Source: CAD feature listing. Evaluate the final solid. Frame: model axes, mm. A direction names the side the tool comes from. Coordinates: 2 decimals unless noted, no trailing zeros. Order: outer loops, then holes, each group sorted by start corner. A loop starts at its lowest first (then second) coordinate and runs counter-clockwise, first axis right, second up.
```python
from build123d import *

# Parameters (mm, degrees)
SKETCH1_W           = 340
SKETCH1_H           = 198
BOSS_EXTRUDE1_DEPTH = 22


with BuildPart() as part:
    # Sketch1 → Boss-Extrude1 (new body)
    with BuildSketch(Plane.XY):
        Polygon((-217.5, 109), (217.5, 109), (217.5, 99), (180, 99), (180, -109), (-180, -109), (-180, 99), (-217.5, 99), align=None)
        Rectangle(SKETCH1_W, SKETCH1_H, mode=Mode.SUBTRACT)
    extrude(amount=BOSS_EXTRUDE1_DEPTH)


solid = part.part
```
1. Section query C-C on y = -17. Return loops of the section in (x, z), plus the area to 3 significant figures.
Findings:
outline: (-180, 0) - (-170, 0) - (-170, 22) - (-180, 22) - close; (170, 0) - (180, 0) - (180, 22) - (170, 22) - close
area: 440 mm2
2. Access query for faces 1 (the face through (-198, 99, 11)), 2 (the face through (180, -4, 11)), 3 (the face through (170, -1, 11)), 4 (the face through (217.5, 104, 11)). Directions: +Z, -Z, +X, -X, +Y, -Y. A direction counts if a zero-diameter tool reaches every point of the face in a straight line with its end or side. Return the directions, or none.
Findings:
face 1: +Z, -Z, -X, -Y
face 2: +Z, -Z, +X, -Y
face 3: +Z, -Z
face 4: +Z, -Z, +X, +Y, -Y
3. Pin query (flat end, axial travel): P1, Ø11, axis at x = 192.5, z = 9.5, coming from the -Y side; P2, Ø4, axis at y = 73, z = 13.5, coming from the +X side; P3, Ø4, axis at y = 11.5, z = 14, coming from the -X side. Return the tip coordinate at first contact, or that it passes through.
Findings:
P1: stops at y = 99
P2: stops at x = 180
P3: stops at x = -180
4. Draft query along Y for faces 5 (the face through (-2, 99, 11)), 6 (the face through (3, -109, 11)), 7 (the face through (-217.5, 104, 11)). Return one class per face: released by +Y, released by -Y, zero draft, split by the parting line, or undercut.
Findings:
face 5: undercut
face 6: released by -Y
face 7: zero draft
5. Section query B-B on z = 6. Return loops of the section in (x, y), plus the area to 3 significant figures.
Findings:
outline: (-217.5, 99) - (-180, 99) - (-180, -109) - (180, -109) - (180, 99) - (217.5, 99) - (217.5, 109) - (-217.5, 109) - close; hole (-170, -99) - (170, -99) - (170, 99) - (-170, 99) - close
area: 11,900 mm2
6. Section query D-D on x = -187. Return loops of the section in (y, z).
Findings:
outline: (99, 0) - (109, 0) - (109, 22) - (99, 22) - close
7. Section query A-A on x = 51.5. Return loops of the section in (y, z), plus the area to 3 significant figures.
Findings:
outline: (-109, 0) - (-99, 0) - (-99, 22) - (-109, 22) - close; (99, 0) - (109, 0) - (109, 22) - (99, 22) - close
area: 440 mm2
8. Ray query, line 1 (X direction, y = 20.5, z = 18); line 2 (Y direction, x = -123.5, z = 6.5); line 3 (Y direction, x = -187, z = 15.5). Return the intervals inside material, ascending.
Findings:
line 1: x = -180 to -170, 170 to 180
line 2: y = -109 to -99, 99 to 109
line 3: y = 99 to 109
